Can you work these out from the model? Positions are in its coordinate system, mm. Face numbers are marked on the shaded views. A direction names the side the tool comes from. Coordinates: 2 decimals unless noted, no trailing zeros. Order: outer loops, then holes, each group sorted by start corner. A loop starts at its lowest first (then second) coordinate and runs counter-clockwise, first axis right, second up. Notation, with made-up numbers: (18, 38) -> (38, 38) arc R17 cw to (38, 66) -> close; hole circle Ø3 at (22, 29). An arc over 180 degrees is marked (long way). Answer in a Markdown table with one row per item. Add a question column.
1. Imagine slicing it at D-D on z = -27.5. Write out the boundary of the cut face in (x, y).
2. On a 3-axis mill with a long thin cutter (end or side, diameter ignored), from which of +Z, -Z, +X, -X, +Y, -Y can I reach the whole of each face in a straight line? I mean the marked faces 5, 6, 7 and 8. Say none if no direction works.
3. If I drill on line 1 along Z through (x, y) = (-20, 5.25); line 2 along Y through (x, z) = (-20, -36.25); line 3 along Z through (x, y) = (-49.5, 28.5), over which ranges is the centre line in solid material (lowest first)? Write a range as [from, to].
4. Imagine slicing it at B-B on z = -35. Write out the boundary of the cut face in (x, y), plus the area to 3 significant figures.
5. Will these pins go through, and if not, where does the flat tip stop? pin 1 (8 mm diameter, centred on x = -20, z = -20, fed in from -Y) (3 decimals); pin 2 (10 mm diameter, centred on x = -39.5, y = 19, fed in from +Z); pin 3 (12 mm diameter, centred on x = -93, z = -42.5, fed in from +Y); pin 4 (18 mm diameter, centred on x = -11.5, y = 45.5, fed in from -Z).
6. We'd pull the mould along Z, two halves only. Please class the marked faces 1, 2, 3 and 4: pulls with the +Z half, pulls with the -Z half, needs draft (parallel to the pull), parting line crosses it, or undercut.
7. Imagine slicing it at A-A on x = -60. Write out the boundary of the cut face in (y, z), plus the area to 3 significant figures.
8. Imagine slicing it at C-C on y = 3.5. Write out the boundary of the cut face in (x, z).
Autodesk Inventor part; units mm, degrees
ref_plane "YZ Plane" through (0, 0, 0) normal (1, 0, 0) x (0, 1, 0)
ref_plane "XZ Plane" through (0, 0, 0) normal (0, 1, 0) x (-1, 0, 0)
ref_plane "XY Plane" through (0, 0, 0) normal (0, 0, 1) x (1, 0, 0)
sketch "Boceto1" plane through (0, 0, 0) normal (0, 1, 0) x (-1, 0, 0)
  line L0 (20, 0) -> (120, 0)
  line L1 (120, 0) -> (120, -70)
  line L2 (120, -70) -> (20, -70)
  line L3 (0, -50) -> (0, -20)
  arc A0 (20, 0) -> (0, -20) centre (20, -20) ccw
  arc A1 (0, -50) -> (20, -70) centre (20, -50) ccw
  circle A2 centre (20, -20) radius 5
  circle A3 centre (20, -50) radius 5
  line L4 (120, -35) -> (60, -35)
  line L5 (120, -35) -> (180, -35) construction
  circle A4 centre (60, -35) radius 15
  circle A5 centre (60, -35) radius 25
  line L6 (120, -39.9519) -> (120, -29.9405)
  line L7 (120, -30) -> (155.5051, -30) construction
  line L8 (120, -40) -> (155.5051, -40) construction
  line L9 (120, -40) -> (84.4949, -40)
  line L10 (35.5051, -40) -> (0, -40)
  line L11 (120, -30) -> (84.4949, -30)
  line L12 (35.5051, -30) -> (0, -30)
  point P0 (0, 0)
  point P1 (0, -70)
  dimension "d0" = 120
  dimension "d1" = 70
  dimension "d2" = 20
  dimension "d3" = 20
  dimension "d4" = 10
  dimension "d5" = 10
  dimension "d6" = 60
  dimension "d7" = 180
  dimension "d8" = 30
  dimension "d9" = 50
extrude "Extrusión1" add sketch "Boceto1" along normal blind 10 contours L0 L1 L11 A5 L12 L3 A0 | L10 A5 L9 L1 L2 A1 L3
extrude "Extrusión2" add sketch "Boceto1" along normal blind 60 contours L12 A5 L10 L3 | L1 L4 A5 L11 | A5 | L1 L9 A5 L4
fillet "Empalme1" radius 20 1 edges at (0, 60, -35)
sketch "Boceto2" plane through (-120, 10, -30) normal (0, 0, 1) x (1, 0, 0)
  line L0 (35.5051, 0) -> (84.4949, 0)
  line L1 (35.5051, 0) -> (35.5051, 30)
  line L2 (0, 0) -> (100, 0)
  line L3 (35.5051, 30) -> (0, 0)
  line L4 (35.5051, 30) -> (70.5051, 30)
  line L5 (70.5051, 30) -> (70.5051, 50)
  line L6 (84.4949, 50) -> (35.5051, 50)
  line L7 (35.5051, 30) -> (35.5051, 50)
  line L8 (35.5051, 50) -> (0, 50)
  line L9 (0, 50) -> (0, 0)
  line L10 (70.5051, 30) -> (70.5051, 50)
  line L11 (84.4949, 50) -> (35.5051, 50)
  line L12 (35.5051, 50) -> (35.5051, 30)
  line L13 (0, 0) -> (35.5051, 30)
  line L14 (70.5051, 30) -> (35.5051, 30)
  line L15 (70.5051, 30) -> (70.5051, 50)
  line L16 (70.5051, 50) -> (0, 50)
  line L17 (0, 50) -> (0, 0)
  dimension "d17" = 30
  dimension "d18" = 35
  dimension "d19" = 20
extrude "Extrusión4" cut sketch "Boceto2" along normal mid plane 60 contours L7 L6 L5 L4 | L3 L9 L8 L7
sketch "Boceto3" plane through (-35.5051, 10, -30) normal (0, 0, 1) x (1, 0, 0)
  line L0 (35.5051, 0) -> (35.5051, 30)
  line L1 (35.5051, 0) -> (15.5051, 0)
  line L2 (35.5051, 0) -> (15.5051, 0)
  line L3 (15.5051, 0) -> (15.5051, 30)
  circle A0 centre (15.5051, 30) radius 5
  point P0 (35.5051, -10)
  dimension "d25" = 10
extrude "Extrusión5" cut sketch "Boceto3" against normal blind 60
sketch "Boceto4" plane through (0, 0, 0) normal (0, -1, 0) x (1, 0, 0)
  line L0 (-120, -30) -> (-120, 0)
  line L1 (-120, 0) -> (-100, 0)
  line L2 (-100, 0) -> (-100, -10)
  line L3 (-100, -10) -> (-120, -10)
  line L4 (-120, -10) -> (-120, 0)
  line L5 (-120, -60.1296) -> (-100, -60.1296)
  line L6 (-100, -60.1296) -> (-100, -70.1296)
  line L7 (-100, -70.1296) -> (-120, -70.1296)
  line L8 (-120, -70.1296) -> (-120, -60.1296)
  line L9 (-100, -10) -> (-100, -60.1296)
  line L10 (-120, -10) -> (-120, -60.1296)
  point P0 (0, 0)
  dimension "d28" = 20
  dimension "d29" = 10
  dimension "d30" = 20
  dimension "d31" = 10
extrude "Extrusión6" add sketch "Boceto4" along normal blind 10 contours L0 L3 L9 L5 L10
extrude "Extrusión7" add sketch "Boceto4" along normal blind 20 contours L0 L1 L2 L3 | L5 L6 L7 L8
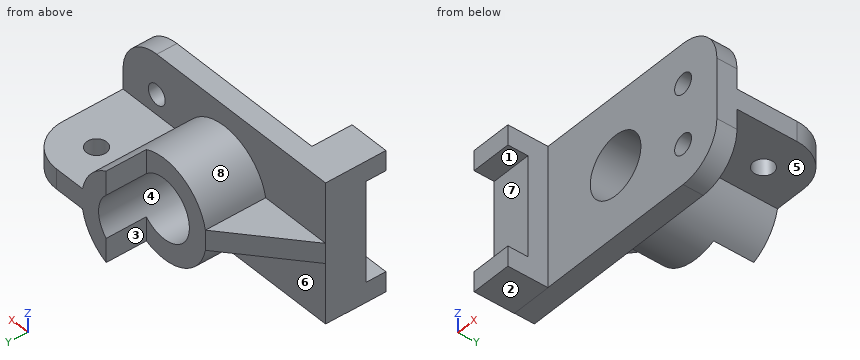
Answers follow:
| question | item | result |
|---|---|---|
| 1 | outline | (-120, -10) -> (-100, -10) -> (-100, 0) -> (-72.99, 0) -> (-72.99, 40) -> (-83.85, 40) -> (-83.85, 10) -> (-120, 10) -> close; (-47.01, 0) -> (0, 0) -> (0, 10) -> (-36.15, 10) -> (-36.15, 60) -> (-47.01, 60) -> close |
| 2 | face 5 | -Z, +X, +Y |
| 2 | face 6 | -Z, +Y |
| 2 | face 7 | +X, -X, -Y |
| 2 | face 8 | +Z, +Y |
| 3 | line 1 | z = [-70, -55], [-45, -25], [-15, 0] |
| 3 | line 2 | y = [0, 35], [45, 60] |
| 3 | line 3 | z = [-57.69, -45.71], [-24.29, -12.31] |
| 4 | outline | (-120, -10) -> (-100, -10) -> (-100, 0) -> (-75, 0) -> (-75, 40) -> (-84.49, 40) -> (-120, 10) -> close; (-45, 0) -> (0, 0) -> (0, 40) arc R20 ccw to (-20, 60) -> (-45, 60) -> close; hole circle Ø10 at (-20, 40) |
| 4 | area | 4,000 mm² |
| 5 | pin 1 | passes through |
| 5 | pin 2 | stops at z = -15.38 |
| 5 | pin 3 | stops at y = 37.42 |
| 5 | pin 4 | stops at z = -40 |
| 6 | face 1 | undercut |
| 6 | face 2 | pulls with the -Z half |
| 6 | face 3 | needs draft |
| 6 | face 4 | undercut |
| 7 | outline | (0, -70) -> (10, -70) -> (10, -60) -> (40, -60) -> (40, -50) -> (0, -50) -> close; (0, -20) -> (40, -20) -> (40, -10) -> (10, -10) -> (10, 0) -> (0, 0) -> close |
| 7 | area | 1,000 mm² |
| 8 | outline | (-120, -70) -> (-20, -70) arc R20 ccw to (0, -50) -> (0, -20) arc R20 ccw to (-20, 0) -> (-120, 0) -> close; hole circle Ø30 at (-60, -35); hole circle Ø10 at (-20, -50); hole circle Ø10 at (-20, -20) |
